Geometry check sheet. Reference: the model listing, model coordinates, mm. A direction names the side the tool comes from. Round coordinates to 2 decimals unless told otherwise and drop trailing zeros. Order: outer loops, then holes, each group sorted by start corner. A loop starts at its lowest first (then second) coordinate and runs counter-clockwise, first axis right, second up.
```python
from build123d import *

# Parameters (mm, degrees)
F1_DEPTH = 7.9375
F2_R     = 3.175
F3_DEPTH = 11.43
F4_R     = 1.5875
F5_DEPTH = 10.16


with BuildPart() as f1:
    # F0 (on Front) → F1 (new body)
    with BuildSketch(Plane.XZ):
        with BuildLine():
            Line((-1.7748789571, 0), (1.7748789571, 0))
            ThreePointArc((1.7748789571, 0), (2.38125, 1.5875), (1.7748789571, 3.175))
            Line((1.7748789571, 3.175), (-1.7748789571, 3.175))
            ThreePointArc((-1.7748789571, 3.175), (-2.38125, 1.5875), (-1.7748789571, 0))
        make_face()
    extrude(amount=-F1_DEPTH)

    # F2 (on face) → F3 (join)
    with BuildSketch(Plane.XZ):
        with Locations((0, 1.5875)):
            Circle(F2_R)
        with BuildLine():
            Line((-1.7748789571, 3.175), (1.7748789571, 3.175))
            ThreePointArc((1.7748789571, 3.175), (2.38125, 1.5875), (1.7748789571, 0))
            Line((1.7748789571, 0), (-1.7748789571, 0))
            ThreePointArc((-1.7748789571, 0), (-2.38125, 1.5875), (-1.7748789571, 3.175))
        make_face(mode=Mode.SUBTRACT)
        with BuildLine():
            ThreePointArc((1.7748789571, 0), (2.38125, 1.5875), (1.7748789571, 3.175))
            Line((1.7748789571, 3.175), (-1.7748789571, 3.175))
            ThreePointArc((-1.7748789571, 3.175), (-2.38125, 1.5875), (-1.7748789571, 0))
            Line((-1.7748789571, 0), (1.7748789571, 0))
        make_face()
    extrude(amount=F3_DEPTH)

    # F4 (on face) → F5 (cut)
    with BuildSketch(Plane.XZ.offset(11.43)):
        with Locations((0, 1.5875)):
            Circle(F4_R)
    extrude(amount=-F5_DEPTH, mode=Mode.SUBTRACT)


solid = f1.part
```
(1) Draft check along X on faces 4 (the cylindrical face through (3.03, -5.63, 2.54)), 5 (the cylindrical face through (-0.21, -6.42, 3.16)), 6 (the flat face through (1, -11.43, 0)), 7 (the flat face through (0, -1.27, 2)). Enter one of: released by +X, released by -X, zero draft, split by the parting line, or undercut.
Returned:
face 4: split by the parting line
face 5: undercut
face 6: zero draft
face 7: undercut
(2) Sectioned sample at C-C, the plane z = 3. Record the cut outline in (x, y).
Returned:
outline: (-2.84, -11.43) - (-0.72, -11.43) - (-0.72, -1.27) - (0.72, -1.27) - (0.72, -11.43) - (2.84, -11.43) - (2.84, 0) - (1.92, 0) - (1.92, 7.94) - (-1.92, 7.94) - (-1.92, 0) - (-2.84, 0) - close
(3) Depth check by flat-ended pin: P1, Ø2, axis at y = 5, z = -0.5, coming from the +X side; P2, Ø1.6, axis at x = 0, z = 1.5, coming from the -Y side; P3, Ø1.8, axis at x = 1, y = 5, coming from the -Z side. Enter the tip coordinate at first touch or a pass-through.
Returned:
P1: stops at x = 2.12
P2: stops at y = -1.27
P3: stops at z = 0
(4) Set-up check for faces 1 (the flat face through (0, 0, -0.5)), 2 (the cylindrical face through (2.38, 3.91, 1.56)), 3 (the cylindrical face through (-2.38, 3.91, 1.61)): record each of +Z, -Z, +X, -X, +Y, -Y from which the full face is reachable in a straight line by a thin tool's end or side.
Returned:
face 1: +Y
face 2: +X, +Y
face 3: -X, +Y
(5) Sectioned sample at D-D, the plane y = 0.5. Record the cut outline in (x, z) (1 decimal), and give its area (3 significant figures).
Returned:
outline: (-1.8, 0) - (1.8, 0) arc R2.4 ccw to (1.8, 3.2) - (-1.8, 3.2) arc R2.4 ccw to start
area: 13.9 mm2
(6) Material ranges on line 1 (Z direction, x = 0, y = -5.5) (1 decimal); line 2 (Y direction, x = 1.75, z = 4); line 3 (X direction, y = -3, z = 1), recorded low to high.
Returned:
line 1: z = -1.6 to 0, 3.2 to 4.8
line 2: y = -11.43 to 0
line 3: x = -3.12 to -1.47, 1.47 to 3.12
(7) Sectioned sample at A-A, the plane x = 0. Record the cut outline in (y, z) (1 decimal).
Returned:
outline: (-11.4, -1.6) - (0, -1.6) - (0, 0) - (7.9, 0) - (7.9, 3.2) - (0, 3.2) - (0, 4.8) - (-11.4, 4.8) - (-11.4, 3.2) - (-1.3, 3.2) - (-1.3, 0) - (-11.4, 0) - close
